Design review of the part built by this model. Coordinates are the model's own, in mm. Round coordinates to 2 decimals unless told otherwise and drop trailing zeros. Loops run counter-clockwise (first coordinate to the right, second up) from the corner with the lowest first, then second, coordinate; pieces in that order, holes last. Notation, with made-up numbers: (-34, -33) - (-18, -33) arc R26 cw to (-18, -18) - close; hole circle Ø5 at (-12.75, 31). An arc over 180 degrees is marked (long way). Answer as CSV lines item,"result". Start each with the question number.
(1) For P1, Ø1, axis at x = 30.5, z = -4, coming from the -Y side; P2, Ø4, axis at x = 62, z = -7.5, coming from the +Y side; P3, Ø1.2, axis at x = 27.5, y = 1.5, coming from the +Z side, all flat-tipped, find the tip position at first contact; note any pin that passes through.
(2) Consider section C-C (x = 54.5). Give the boundary of the cut face in (y, z).
(3) Consider section B-B (z = -10). Give the boundary of the cut face in (x, y).
(4) Consider section A-A (z = 13.5). Give the boundary of the cut face in (x, y), and give its area (3 significant figures).
(5) Wall thickness on L1, parallel to X at y = 0.5, z = 17.5; L2, parallel to Z at x = 41, y = 1.2; L3, parallel to X at y = 2.7, z = 6: over which ranges is each line inside the solid? List them lowest first.
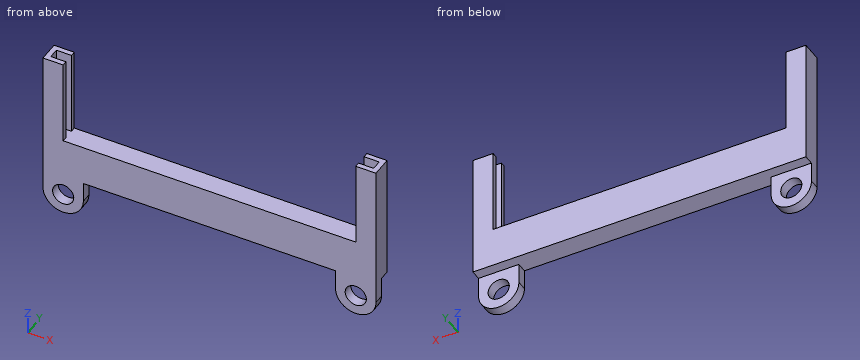
Autodesk Inventor part; units mm, degrees
ref_plane "Work Plane1" through (0, 0, 20) normal (0, 0, 1) x (1, 0, 0)
ref_plane "YZ Plane" through (0, 0, 0) normal (1, 0, 0) x (0, 1, 0)
ref_plane "XZ Plane" through (0, 0, 0) normal (0, 1, 0) x (-1, 0, 0)
sketch "Sketch1" plane through (0, 0, 0) normal (0, 0, 1) x (1, 0, 0)
  line L0 (0, 0) -> (66, 0)
  line L1 (66, 0) -> (66, 4)
  line L2 (66, 4) -> (0, 4)
  line L3 (0, 4) -> (0, 0)
  dimension "d0" = 66
  dimension "d1" = 4
extrude "Extrusion1" add sketch "Sketch1" along normal blind 20
sketch "Sketch2" plane through (0, 4, 0) normal (0, 1, 0) x (1, 0, 0)
  line L0 (0, -20) -> (66, -20)
  line L1 (4, -20) -> (62, -20)
  line L2 (62, -20) -> (62, -3)
  line L3 (62, -3) -> (4, -3)
  line L4 (4, -3) -> (4, -20)
  line L5 (0, 0) -> (0, -20)
  dimension "d4" = 58
  dimension "d5" = 17
  dimension "d6" = 4
extrude "Extrusion2" cut sketch "Sketch2" against normal blind 20
ref_plane "Work Plane1" through (0, 0, 20) normal (0, 0, 1) x (1, 0, 0)
sketch "Sketch3" plane through (0, 0, 20) normal (0, 0, 1) x (1, 0, 0)
  line L0 (4, 0) -> (4, 4)
  line L1 (4, 4) -> (0, 4)
  line L2 (0, 4) -> (0, 0)
  line L3 (0, 0) -> (4, 0)
  line L4 (62, 4) -> (62, 0)
  line L5 (62, 0) -> (66, 0)
  line L6 (66, 0) -> (66, 4)
  line L7 (66, 4) -> (62, 4)
  line L8 (4, 0) -> (1, 0)
  line L9 (4, 1) -> (4, 0)
  line L10 (1, 3) -> (4, 3)
  line L11 (4, 3) -> (4, 1)
  line L12 (4, 1) -> (1, 1)
  line L13 (1, 1) -> (1, 3)
  line L14 (62, 3) -> (65, 3)
  line L15 (65, 3) -> (65, 1)
  line L16 (65, 1) -> (62, 1)
  line L17 (62, 1) -> (62, 3)
  dimension "d30" = 3
  dimension "d31" = 2
  dimension "d32" = 1
  dimension "d33" = 4
  dimension "d34" = 3
  dimension "d35" = 2
  dimension "d36" = 1
  dimension "d37" = 4
extrude "Extrusion3" cut sketch "Sketch3" against normal blind 17 contours L12 L13 L10 L0 | L14 L15 L16 L4
sketch "Sketch4" plane through (0, 4, 0) normal (0, 1, 0) x (1, 0, 0)
  line L0 (0, 0) -> (66, 0)
  line L1 (60, 5) -> (10, 5)
  line L2 (0, 5) -> (0, 0)
  line L3 (60, 5) -> (66, 5)
  line L4 (60, 5) -> (0, 5)
  line L5 (4, -20) -> (4, -3)
  line L6 (4, -3) -> (62, -3)
  line L7 (62, -3) -> (62, -20)
  line L8 (66, -20) -> (62, -20)
  line L9 (66, 0) -> (66, -20)
  line L10 (66, 0) -> (0, 0)
  line L11 (0, 0) -> (0, -20)
  line L12 (4, -20) -> (0, -20)
  line L13 (66, 0) -> (66, 5)
  point P0 (66.0117, 5)
extrude "Extrusion5" add sketch "Sketch4" against normal blind 4 contours L2 L4 L1 L3 L13 L0
sketch "Sketch6" plane through (4, 0, 3) normal (0, -1, 0) x (1, 0, 0)
  circle A0 centre (58, -12) radius 2.1
  arc A1 (54, -12) -> (62, -12) centre (58, -12) ccw
  line L0 (54, -12) -> (54, -8)
  arc A2 (-4, -12) -> (4, -12) centre (0, -12) ccw
  circle A3 centre (0, -12) radius 2.1
  line L1 (4, -12) -> (4, -8)
  line L2 (-4, -12) -> (-4, -8)
  line L3 (62, -8) -> (62, 17)
  line L4 (62, -8) -> (-4, -8)
  line L5 (62, -8) -> (62, 17)
  line L6 (62, -8) -> (62, -12)
  line L7 (-4, 17) -> (-4, -8)
  dimension "d40" = 4.2
  dimension "d41" = 8
  dimension "d44" = 8
  dimension "d45" = 4.2
  dimension "d53" = 4
  dimension "d54" = 4
  dimension "d55" = 4
  dimension "d56" = 4
extrude "Extrusion6" add sketch "Sketch6" against normal blind 2
properties part number "Electronics-Wedge"
Determined:
1,P1,"stops at y = 0"
1,P2,"stops at y = 2"
1,P3,"stops at z = 3"
2,outline,"(0, -5) - (4, -5) - (4, 3) - (0, 3) - close"
3,outline,"(0.13, 0) - (2.15, 0) - (2.15, 2) - (0.13, 2) - close; (5.85, 0) - (7.87, 0) - (7.87, 2) - (5.85, 2) - close; (58.13, 0) - (60.15, 0) - (60.15, 2) - (58.13, 2) - close; (63.85, 0) - (65.87, 0) - (65.87, 2) - (63.85, 2) - close"
4,outline,"(0, 0) - (4, 0) - (4, 1) - (1, 1) - (1, 3) - (4, 3) - (4, 4) - (0, 4) - close; (62, 0) - (66, 0) - (66, 4) - (62, 4) - (62, 3) - (65, 3) - (65, 1) - (62, 1) - close"
4,area,"20.0 mm^2"
5,L1,"x = 0 to 4, 62 to 66"
5,L2,"z = -5 to 3"
5,L3,"x = 0 to 1, 65 to 66"
